from build123d import *

# Parameters (mm, degrees)
SKETCH1_W           = 44.2
SKETCH1_H           = 24
SKETCH1_W_2         = 40.2
SKETCH1_H_2         = 20
BOSS_EXTRUDE1_DEPTH = 11
SKETCH2_W           = 44.2
SKETCH2_H           = 24
BOSS_EXTRUDE2_DEPTH = 2
SKETCH3_W           = 11
SKETCH3_H           = 8
CUT_EXTRUDE1_DEPTH  = 2
SKETCH4_R           = 2
BOSS_EXTRUDE3_DEPTH = 7
SKETCH5_R           = 0.9
CUT_EXTRUDE2_DEPTH  = 10
SKETCH6_W           = 44.2
SKETCH6_H           = 11
CUT_EXTRUDE3_DEPTH  = 100
SKETCH7_R           = 2.1
CUT_EXTRUDE4_DEPTH  = 1


with BuildPart() as part:
    # Sketch1 → Boss-Extrude1 (new body)
    with BuildSketch(Plane.XY):
        with Locations((20.1, 10)):
            Rectangle(SKETCH1_W, SKETCH1_H)
        with Locations((20.1, 10)):
            Rectangle(SKETCH1_W_2, SKETCH1_H_2, mode=Mode.SUBTRACT)
    extrude(amount=BOSS_EXTRUDE1_DEPTH)

    # Sketch2 → Boss-Extrude2 (add)
    with BuildSketch(Plane.XY.offset(11)):
        with Locations((20.1, 10)):
            Rectangle(SKETCH2_W, SKETCH2_H)
    extrude(amount=BOSS_EXTRUDE2_DEPTH)

    # Sketch3 → Cut-Extrude1 (cut)
    with BuildSketch(Plane(origin=(42.2, 0, 0), x_dir=(0, 0, -1), z_dir=(1, 0, 0))):
        with Locations((-7.5, 10)):
            Rectangle(SKETCH3_W, SKETCH3_H)
    extrude(amount=-CUT_EXTRUDE1_DEPTH, mode=Mode.SUBTRACT)

    # Sketch4 → Boss-Extrude3 (add)
    with BuildSketch(Plane.XY.offset(13)):
        with Locations((32.32, 10)):
            Circle(SKETCH4_R)
    extrude(amount=BOSS_EXTRUDE3_DEPTH)

    # Sketch5 → Cut-Extrude2 (cut)
    with BuildSketch(Plane(origin=(0, 0, 11), x_dir=(-1, 0, 0), z_dir=(0, 0, -1))):
        with Locations((-38.4, 18.2)):
            Circle(SKETCH5_R)
        with Locations(Location((-1.8, 18.2, 0), (0, 0, 180))):
            Circle(SKETCH5_R)
        with Locations((-1.8, 1.8)):
            Circle(SKETCH5_R)
        with Locations(Location((-38.4, 1.8, 0), (0, 0, 180))):
            Circle(SKETCH5_R)
    extrude(amount=-CUT_EXTRUDE2_DEPTH, mode=Mode.SUBTRACT)

    # Sketch6 → Cut-Extrude3 (cut)
    with BuildSketch(Plane(origin=(0, 22, 0), x_dir=(1, 0, 0), z_dir=(0, 1, 0))):
        with Locations((20.1, -5.5)):
            Rectangle(SKETCH6_W, SKETCH6_H)
    extrude(amount=-CUT_EXTRUDE3_DEPTH, mode=Mode.SUBTRACT)

    # Sketch7 → Cut-Extrude4 (cut)
    with BuildSketch(Plane.XY.offset(13)):
        with Locations((1.8, 18.2)):
            Circle(SKETCH7_R)
        with Locations((38.4, 18.2)):
            Circle(SKETCH7_R)
        with Locations((38.4, 1.8)):
            Circle(SKETCH7_R)
        with Locations((1.8, 1.8)):
            Circle(SKETCH7_R)
    extrude(amount=-CUT_EXTRUDE4_DEPTH, mode=Mode.SUBTRACT)


solid = part.part
Geometry: final body of the model. Coordinates: model frame, mm. A direction names the side the tool comes from. Round coordinates to 2 decimals unless told otherwise and drop trailing zeros. Loops run counter-clockwise (first coordinate to the right, second up) from the corner with the lowest first, then second, coordinate; pieces in that order, holes last. Notation, with made-up numbers: M -29.75,22.25 L -5.75,22.25 A26 ccw -5.75,40.25 Z; hole C 23.25,53 d5. An arc over 180 degrees is marked long. One line per question, with ' | ' between items.
(1) Cut plane C-C on y = 10. Return the cut outline in (x, z), plus the area to 3 significant figures.
Check result:
outline: M -2,11 L 40.2,11 L 40.2,13 L 34.32,13 L 34.32,20 L 30.32,20 L 30.32,13 L -2,13 Z | area: 112 mm2
(2) Material intervals for line 1 along Y through (x, z) = (1.8, 11.65); line 2 along Y through (x, z) = (1.8, 12.55); line 3 along Z through (x, y) = (28.5, 17.5), sorted ascending. Write a range as from..to.
Check result:
line 1: y = -2..0.9, 2.7..17.3, 19.1..22 | line 2: y = -2..-0.3, 3.9..16.1, 20.3..22 | line 3: z = 11..13
(3) Contact query for flat-ended pins moving along their axis: P1, Ø3, axis at y = 8, z = 16, coming from the -X side; P2, Ø2, axis at x = 38.4, y = 1.8, coming from the +Z side; P3, Ø2, axis at x = 3.5, y = 15, coming from the +Z side. Output: stop coordinate, or through.
Check result:
P1: stops at x = 30.38 | P2: stops at z = 12 | P3: stops at z = 13
(4) Cut plane A-A on y = 18.2. Return the cut outline in (x, z), plus the area to 3 significant figures.
Check result:
outline: M -2,11 L 0.9,11 L 0.9,12 L -0.3,12 L -0.3,13 L -2,13 Z; M 2.7,11 L 37.5,11 L 37.5,12 L 36.3,12 L 36.3,13 L 3.9,13 L 3.9,12 L 2.7,12 Z; M 39.3,11 L 42.2,11 L 42.2,13 L 40.5,13 L 40.5,12 L 39.3,12 Z | area: 76.4 mm2
(5) Pull-direction query (X, two-part tool) for faces 1 (the flat face through (20, 10, 13)), 2 (the flat face through (42.2, 2, 12)), 3 (the cylindrical face through (39.53, 19.97, 12.51)), 4 (the flat face through (38, 17, 12)); classes: +X half, -X half, draft (parallel to the pull), parting line (faces both ways), or undercut.
Check result:
face 1: draft | face 2: +X half | face 3: undercut | face 4: undercut
(6) Access query for faces 5 (the flat face through (41, 14, 12)), 6 (the cylindrical face through (0.252, 3.219, 12.507)), 7 (the flat face through (42.2, 18, 12)). Directions: +Z, -Z, +X, -X, +Y, -Y. A direction counts if a zero-diameter tool reaches every point of the face in a straight line with its end or side. Return the directions, or none.
Check result:
face 5: +Z, -Z, +X | face 6: +Z | face 7: +Z, -Z, +X, +Y, -Y
(7) Cut plane B-B on x = 38.4. Return the cut outline in (y, z).
Check result:
outline: M -2,11 L 0.9,11 L 0.9,12 L -0.3,12 L -0.3,13 L -2,13 Z; M 2.7,11 L 17.3,11 L 17.3,12 L 16.1,12 L 16.1,13 L 3.9,13 L 3.9,12 L 2.7,12 Z; M 19.1,11 L 22,11 L 22,13 L 20.3,13 L 20.3,12 L 19.1,12 Z
(8) Cut plane D-D on z = 15.25. Return the cut outline in (x, y).
Check result:
outline: C 32.32,10 d4
